Here's how the part is built. I have some questions about the finished solid (model axes, mm). Face numbers are marked on the shaded views. Give positions to 0.01 mm unless a question says otherwise; leave off trailing zeros. Write each loop counter-clockwise with the first axis right and the second up, starting at its lowest first coordinate (ties: lowest second). Pieces come first, ordered by that corner, then holes. Notation, with made-up numbers: (67.25, 75) - (116.25, 75) arc R6 ccw to (116.25, 79) - close; hole circle Ø1 at (36.25, -23). An arc over 180 degrees is marked (long way). Write each question's results on one line, items separated by ' | '. Start each with the question number.
Item 1: We'd pull the mould along Y, two halves only. Please class the marked faces 1, 2 and 3: +Y half, -Y half, draft (parallel to the pull), parting line (faces both ways), or undercut.
Item 2: Suppose I cut it at B-B on y = 0. List the corners of the cut face in (x, z) for me.
Item 3: Please list where these lines run through material, in increasing order: line 1 along Y through (x, z) = (0, 3.5); line 2 along Y through (x, z) = (-7.5, 0.75); line 3 along X through (y, z) = (-8, 6).
Item 4: Suppose I cut it at C-C on z = 0.5. List the corners of the cut face in (x, y) for me (1 decimal), then the cut area to 3 significant figures.
Item 5: Suppose I cut it at D-D on y = 6. List the corners of the cut face in (x, z) for me.
Item 6: Suppose I cut it at A-A on x = 0. List the corners of the cut face in (y, z) for me.
Item 7: Will these pins go through, and if not, where does the flat tip stop? P1, Ø4, axis at y = 2.5, z = 3.5, coming from the -X side; P2, Ø0.6, axis at x = 16, z = 1, coming from the +Y side; P3, Ø0.9, axis at x = -16, z = 0.5, coming from the -Y side; P4, Ø1.3, axis at x = -16.5, z = 7, coming from the -Y side.
Autodesk Inventor part; units mm, degrees
ref_plane "YZ Plane" through (0, 0, 0) normal (1, 0, 0) x (0, 1, 0)
ref_plane "XZ Plane" through (0, 0, 0) normal (0, 1, 0) x (-1, 0, 0)
ref_plane "XY Plane" through (0, 0, 0) normal (0, 0, 1) x (1, 0, 0)
sketch "Sketch1" plane through (0, 0, 0) normal (0, 0, 1) x (1, 0, 0)
  circle A0 centre (0, 0) radius 15.5575
  dimension "d0" = 31.115
extrude "Extrusion1" add sketch "Sketch1" along normal blind 7.62
sketch "Sketch2" plane through (0, 0, 7.62) normal (0, 0, 1) x (1, 0, 0)
  circle A0 centre (0, 0) radius 14.3891
  dimension "d16" = 28.7782
extrude "Extrusion2" cut sketch "Sketch2" against normal blind 6.35
sketch "Sketch3" plane through (0, 0, 0) normal (0, 0, -1) x (-1, 0, 0)
  circle A0 centre (0, 0) radius 12.7
  dimension "d15" = 25.4
extrude "Extrusion3" cut sketch "Sketch3" against normal blind 5.08
sketch "Sketch4" plane through (0, 0, 7.62) normal (0, 0, 1) x (1, 0, 0)
  line L0 (-14.2875, -3.1369) -> (-16.8275, -3.1369)
  line L1 (-16.8275, -3.1369) -> (-16.8275, 3.1369)
  line L2 (-16.8275, 3.1369) -> (-14.2875, 3.1369)
  line L3 (-14.2875, 3.1369) -> (-14.2875, -3.1369)
  circle A0 centre (0, 0) radius 15.5575
  line L4 (-14.2875, -3.1369) -> (-16.8275, 3.1369) construction
  line L5 (-16.8275, -3.1369) -> (-14.2875, 3.1369) construction
  line L6 (14.2875, -3.1369) -> (16.8275, -3.1369)
  line L7 (16.8275, -3.1369) -> (16.8275, 3.1369)
  line L8 (16.8275, 3.1369) -> (14.2875, 3.1369)
  line L9 (14.2875, 3.1369) -> (14.2875, -3.1369)
  line L10 (14.2875, -3.1369) -> (16.8275, 3.1369) construction
  line L11 (16.8275, -3.1369) -> (14.2875, 3.1369) construction
  point P0 (-15.5575, 0)
  point P1 (15.5575, 0)
  dimension "d7" = 2.54
  dimension "d8" = 6.2738
  dimension "d9" = 2.54
  dimension "d10" = 6.2738
extrude "Extrusion5" add sketch "Sketch4" against normal blind 2.286 contours L0 A0 L2 L3 | L0 L1 L2 A0 | L6 L9 L8 A0 | A0 L8 L7 L6
sketch "Sketch5" plane through (0, 0, 0) normal (0, 0, -1) x (-1, 0, 0)
  line L0 (13.97, 2.3319) -> (16.51, 2.3319)
  line L1 (16.51, 2.3319) -> (16.51, -2.3319)
  line L2 (16.51, -2.3319) -> (13.97, -2.3319)
  line L3 (13.97, -2.3319) -> (13.97, 2.3319)
  line L4 (13.97, 2.3319) -> (16.51, -2.3319) construction
  line L5 (16.51, 2.3319) -> (13.97, -2.3319) construction
  line L6 (-16.51, 2.3319) -> (-13.97, 2.3319)
  line L7 (-13.97, 2.3319) -> (-13.97, -2.3319)
  line L8 (-13.97, -2.3319) -> (-16.51, -2.3319)
  line L9 (-16.51, -2.3319) -> (-16.51, 2.3319)
  line L10 (-16.51, 2.3319) -> (-13.97, -2.3319) construction
  line L11 (-13.97, 2.3319) -> (-16.51, -2.3319) construction
  point P0 (0, 0)
  point P1 (15.24, 0)
  point P2 (-15.24, 0)
  dimension "d17" = 2.54
  dimension "d18" = 2.54
  dimension "d19" = 15.24
  dimension "d20" = 15.24
extrude "Extrusion6" add sketch "Sketch5" against normal blind 1.27
properties part number "GelCupHolderTop"
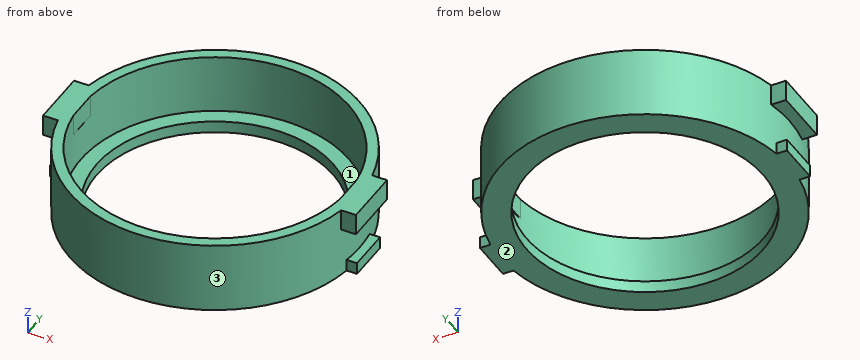
Checked values:
1) face 1: undercut | face 2: draft | face 3: parting line
2) outline: (-16.83, 5.33) - (-15.56, 5.33) - (-15.56, 1.27) - (-16.51, 1.27) - (-16.51, 0) - (-12.7, 0) - (-12.7, 1.27) - (-14.39, 1.27) - (-14.39, 5.33) - (-14.29, 5.33) - (-14.29, 7.62) - (-16.83, 7.62) - close; (12.7, 0) - (16.51, 0) - (16.51, 1.27) - (15.56, 1.27) - (15.56, 5.33) - (16.83, 5.33) - (16.83, 7.62) - (14.29, 7.62) - (14.29, 5.33) - (14.39, 5.33) - (14.39, 1.27) - (12.7, 1.27) - close
3) line 1: y = -15.56 to -14.39, 14.39 to 15.56 | line 2: y = -13.63 to -10.25, 10.25 to 13.63 | line 3: x = -13.34 to -11.96, 11.96 to 13.34
4) outline: (-16.5, -2.3) - (-15.4, -2.3) arc R15.6 ccw to (15.4, -2.3) - (16.5, -2.3) - (16.5, 2.3) - (15.4, 2.3) arc R15.6 ccw to (-15.4, 2.3) - (-16.5, 2.3) - close; hole circle Ø25.4 at (0, 0) | area: 263 mm^2
5) outline: (-14.35, 0) - (-11.19, 0) - (-11.19, 1.27) - (-13.08, 1.27) - (-13.08, 7.62) - (-14.35, 7.62) - close; (11.19, 0) - (14.35, 0) - (14.35, 7.62) - (13.08, 7.62) - (13.08, 1.27) - (11.19, 1.27) - close
6) outline: (-15.56, 0) - (-12.7, 0) - (-12.7, 1.27) - (-14.39, 1.27) - (-14.39, 7.62) - (-15.56, 7.62) - close; (12.7, 0) - (15.56, 0) - (15.56, 7.62) - (14.39, 7.62) - (14.39, 1.27) - (12.7, 1.27) - close
7) P1: stops at x = -16.83 | P2: stops at y = 2.33 | P3: stops at y = -2.33 | P4: stops at y = -3.14
